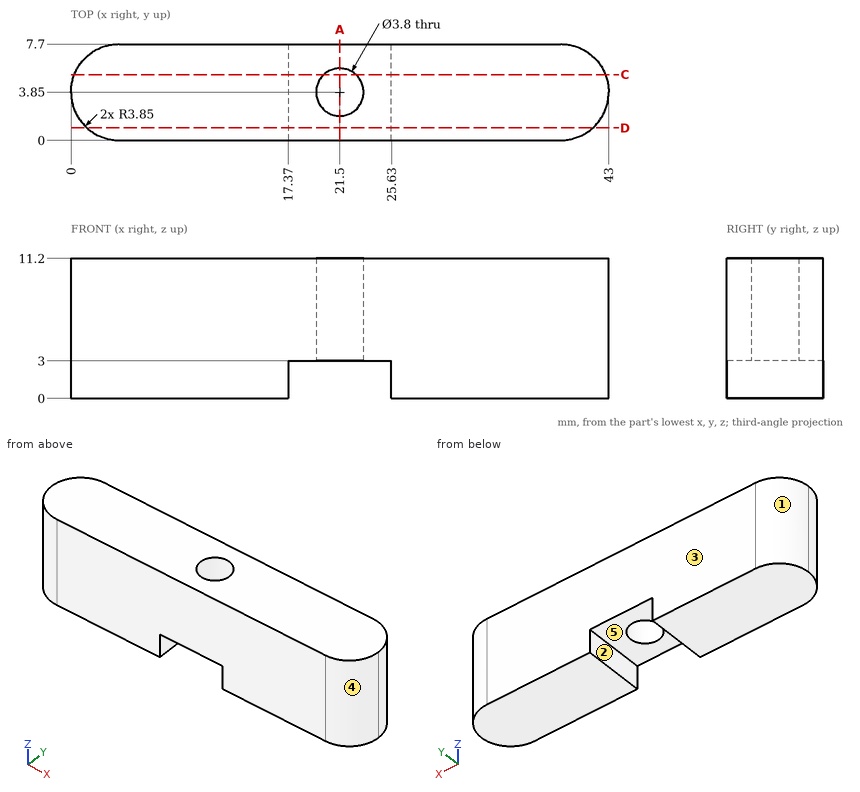
Source: three-view drawing plus pictorial views. Frame: mm from the lowest corner of the part. A direction names the side the tool comes from. Give positions to 0.01 mm unless a question says otherwise; leave off trailing zeros. Order: outer loops, then holes, each group sorted by start corner. A loop starts at its lowest first (then second) coordinate and runs counter-clockwise, first axis right, second up. Notation, with made-up numbers: (-17, -7) -> (23, -7) arc R10 ccw to (23, 1) -> close; hole circle Ø3 at (82, 62). An arc over 180 degrees is marked (long way). Put each result on its own line as item: value.
Q1. Section A-A, the plane x = 21.5. Return loops of the section in (y, z).
Here are the results:
outline: (0, 3) -> (1.95, 3) -> (1.95, 11.2) -> (0, 11.2) -> close; (5.75, 3) -> (7.7, 3) -> (7.7, 11.2) -> (5.75, 11.2) -> close
Q2. Material intervals for L1, parallel to Y at x = 21.5, z = 8.5; L2, parallel to X at y = 4.75, z = 5; L3, parallel to X at y = 5.25, z = 1.5, sorted ascending.
Here are the results:
L1: y = 0 to 1.95, 5.75 to 7.7
L2: x = 0.11 to 19.83, 23.17 to 42.89
L3: x = 0.26 to 17.37, 25.63 to 42.74
Q3. Pin query (flat end, axial travel): pin 1 (3.5 mm diameter, centred on y = 3.5, z = 2, fed in from -X). Return the tip coordinate at first contact, or that it passes through.
Here are the results:
pin 1: stops at x = 0
Q4. Reachability of the marked faces 4 and 5 from +Z, -Z, +X, -X, +Y, -Y: full face, straight path, thin tool, end or side. Return the list, or none.
Here are the results:
face 4: +Z, -Z, +X, -Y
face 5: -Z, +Y, -Y
Q5. Draft query along X for the marked faces 1, 2 and 3. Return one class per face: released by +X, released by -X, zero draft, split by the parting line, or undercut.
Here are the results:
face 1: released by -X
face 2: undercut
face 3: zero draft
Q6. Section D-D, the plane y = 1. Return loops of the section in (x, z), then the cut area to 3 significant figures.
Here are the results:
outline: (1.26, 0) -> (17.37, 0) -> (17.37, 3) -> (25.63, 3) -> (25.63, 0) -> (41.74, 0) -> (41.74, 11.2) -> (1.26, 11.2) -> close
area: 429 mm^2
Q7. Section C-C, the plane y = 5.25. Return loops of the section in (x, z).
Here are the results:
outline: (0.26, 0) -> (17.37, 0) -> (17.37, 3) -> (20.22, 3) -> (20.22, 11.2) -> (0.26, 11.2) -> close; (22.78, 3) -> (25.63, 3) -> (25.63, 0) -> (42.74, 0) -> (42.74, 11.2) -> (22.78, 11.2) -> close
